Autodesk Fusion 360 part; units mm, degrees
sketch "Sketch1" plane through (0, 0, 0) normal (0, 1, 0) x (1, 0, 0)
  line L0 (4.25, 1.85) -> (-4.25, 1.85)
  line L1 (-4.25, 1.85) -> (-4.25, -1.85)
  line L2 (-4.25, -1.85) -> (4.25, -1.85)
  line L3 (4.25, -1.85) -> (4.25, 1.85)
  line L4 (4.25, 1.85) -> (-4.25, -1.85) construction
  line L5 (-4.25, 1.85) -> (4.25, -1.85) construction
  dimension "d1" = 8.5
  dimension "d2" = 3.7
extrude "Extrude1" add sketch "Sketch1" along normal blind 3.3
sketch "Sketch2" plane through (0, 3.3, 0) normal (0, 1, 0) x (-1, 0, 0)
  line L0 (-4.25, 1.85) -> (-4.25, -1.85)
  line L1 (-4.25, -1.85) -> (4.25, -1.85)
  line L2 (4.25, -1.85) -> (4.25, 1.85)
  line L3 (4.25, 1.85) -> (-4.25, 1.85)
  line L4 (-4.25, 0) -> (-1.75, 0)
  line L5 (-1.75, 0) -> (-1.1, 0)
  line L6 (-1.75, -0.65) -> (-0.45, -0.65)
  line L7 (-0.45, -0.65) -> (-0.45, 0.65)
  line L8 (-0.45, 0.65) -> (-1.75, 0.65)
  line L9 (-1.75, 0.65) -> (-1.75, -0.65)
  line L10 (-1.75, -0.65) -> (-0.45, 0.65) construction
  line L11 (-0.45, -0.65) -> (-1.75, 0.65) construction
  line L12 (4.25, 0) -> (1.75, 0)
  line L13 (1.75, 0) -> (1.1, 0)
  line L14 (0.45, -0.65) -> (1.75, -0.65)
  line L15 (1.75, -0.65) -> (1.75, 0.65)
  line L16 (1.75, 0.65) -> (0.45, 0.65)
  line L17 (0.45, 0.65) -> (0.45, -0.65)
  line L18 (0.45, -0.65) -> (1.75, 0.65) construction
  line L19 (1.75, -0.65) -> (0.45, 0.65) construction
  line L20 (0.45, -0.65) -> (-0.45, -0.65)
  line L21 (0.45, 0.65) -> (-0.45, 0.65)
  point P0 (-1.1, 0)
  point P1 (1.1, 0)
  dimension "d5" = 2.5
  dimension "d6" = 0.65
  dimension "d7" = 1.3
  dimension "d8" = 1.3
  dimension "d9" = 2.5
  dimension "d10" = 0.65
  dimension "d11" = 1.3
  dimension "d12" = 1.3
extrude "Extrude2" cut sketch "Sketch2" against normal blind 0.1 contours L14 L15 L16 L17 | L7 L17 L20 L21
extrude "Extrude3" add sketch "Sketch2" along normal blind 3 contours L6 L7 L8 L9
chamfer "Chamfer1" distance 0.2 angle 45 4 edges at (1.1, 6.3, 0.65) (0.45, 6.3, 0) (1.1, 6.3, -0.65) (1.75, 6.3, 0)
chamfer "Chamfer2" distance 0.1 angle 45 12 edges at (0, 3.3, 1.85) (4.25, 3.3, 0) (-4.25, 3.3, 0) (0, 3.3, -1.85) (4.25, 1.65, 1.85) (4.25, 1.65, -1.85) (4.25, 0, 0) (0, 0, 1.85) (-4.25, 1.65, 1.85) (-4.25, 1.65, -1.85) (0, 0, -1.85) (-4.25, 0, 0)
sketch "Sketch3" plane through (0, 0, 0) normal (0, -1, 0) x (1, 0, 0)
  line L0 (-4.15, -1.75) -> (4.15, -1.75)
  line L1 (4.15, -1.75) -> (4.15, 1.75)
  line L2 (4.15, 1.75) -> (-4.15, 1.75)
  line L3 (-4.15, 1.75) -> (-4.15, -1.75)
  line L4 (0.15, 0.1) -> (-0.15, 0.1)
  line L5 (-0.15, 0.1) -> (-0.15, -0.1)
  line L6 (-0.15, -0.1) -> (0.15, -0.1)
  line L7 (0.15, -0.1) -> (0.15, 0.1)
  line L8 (0.15, 0.1) -> (-0.15, -0.1) construction
  line L9 (-0.15, 0.1) -> (0.15, -0.1) construction
  line L10 (0, 0) -> (2.7, 0)
  line L11 (2.7, 0) -> (2.55, 0)
  line L12 (2.7, 0.1) -> (2.4, 0.1)
  line L13 (2.4, 0.1) -> (2.4, -0.1)
  line L14 (2.4, -0.1) -> (2.7, -0.1)
  line L15 (2.7, -0.1) -> (2.7, 0.1)
  line L16 (2.7, 0.1) -> (2.4, -0.1) construction
  line L17 (2.4, 0.1) -> (2.7, -0.1) construction
  line L18 (-0.15, 0) -> (-2.85, 0)
  line L19 (-2.85, 0) -> (-2.7, 0)
  line L20 (-2.55, 0.1) -> (-2.85, 0.1)
  line L21 (-2.85, 0.1) -> (-2.85, -0.1)
  line L22 (-2.85, -0.1) -> (-2.55, -0.1)
  line L23 (-2.55, -0.1) -> (-2.55, 0.1)
  line L24 (-2.55, 0.1) -> (-2.85, -0.1) construction
  line L25 (-2.85, 0.1) -> (-2.55, -0.1) construction
  point P0 (2.55, 0)
  point P1 (-2.7, 0)
  dimension "d19" = 0.3
  dimension "d20" = 0.2
  dimension "d23" = 2.7
  dimension "d24" = 0.15
  dimension "d25" = 0.3
  dimension "d26" = 0.2
  dimension "d27" = 2.7
  dimension "d28" = 0.15
  dimension "d29" = 0.3
  dimension "d30" = 0.2
extrude "Extrude4" add sketch "Sketch3" along normal blind 5 contours L4 L5 L6 L7
extrude "Extrude5" add sketch "Sketch3" along normal blind 5 contours L18 L19 L21 L22 L23 | L18 L19 L20 L21 L23
extrude "Extrude6" add sketch "Sketch3" along normal blind 5 contours L10 L11 L12 L13 L15 | L10 L11 L13 L14 L15
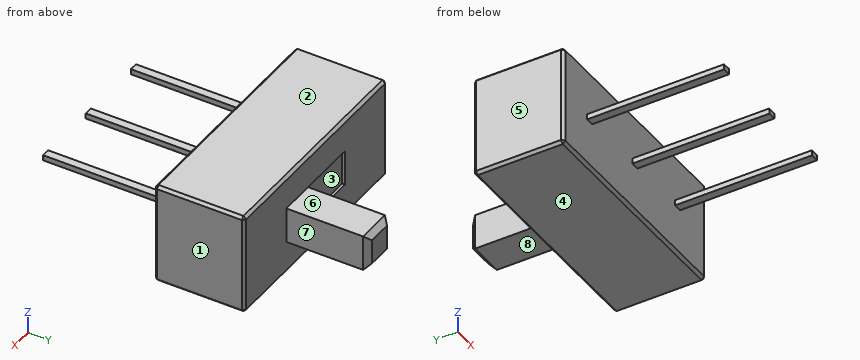
Input: part model. Units: mm. Frame: model coordinates. Face numbers are marked on the shaded views. A direction names the side the tool comes from. Coordinates: 2 decimals unless noted, no trailing zeros. Write each loop counter-clockwise with the first axis right and the second up, starting at its lowest first coordinate (ties: lowest second). Pieces come first, ordered by that corner, then holes. Notation, with made-up numbers: (-24.75, 58) -> (22.25, 58) arc R23 cw to (22.25, 70) -> close; hole circle Ø5 at (-11, -17.5). An arc over 180 degrees is marked (long way). Answer as a JSON object with one key per item and string values.
1. Section D-D on y = 5.25. Return the cut outline in (x, z), then the cut area to 3 significant figures.
Result set:
{"outline": "(0.45, -0.65) -> (1.75, -0.65) -> (1.75, 0.65) -> (0.45, 0.65) -> close", "area": "1.69 mm2"}
2. First-contact query: P1, Ø1, axis at y = 5, z = 0, coming from the +X side; P2, Ø0.6, axis at x = 1, y = 4.5, coming from the +Z side; P3, Ø0.6, axis at x = -0.5, z = 0, coming from the +Y side. Flat tips, straight axial feed; report the tip coordinate or a pass-through.
Result set:
{"P1": "stops at x = 1.75", "P2": "stops at z = 0.65", "P3": "stops at y = 3.2"}
3. Section A-A on y = -3. Return the cut outline in (x, z), then the cut area to 3 significant figures.
Result set:
{"outline": "(-2.85, -0.1) -> (-2.55, -0.1) -> (-2.55, 0.1) -> (-2.85, 0.1) -> close; (-0.15, -0.1) -> (0.15, -0.1) -> (0.15, 0.1) -> (-0.15, 0.1) -> close; (2.4, -0.1) -> (2.7, -0.1) -> (2.7, 0.1) -> (2.4, 0.1) -> close", "area": "0.180 mm2"}
4. Section C-C on z = -0.95. Return the cut outline in (x, y).
Result set:
{"outline": "(-4.25, 0.1) -> (-4.15, 0) -> (4.15, 0) -> (4.25, 0.1) -> (4.25, 3.2) -> (4.15, 3.3) -> (-4.15, 3.3) -> (-4.25, 3.2) -> close"}
5. Mould query, pull axis Z, two halves, no side actions, for the marked faces 1, 2, 3 and 4. Classes: released by +Z, released by -Z, zero draft, split by the parting line, or undercut.
Result set:
{"face 1": "zero draft", "face 2": "released by +Z", "face 3": "undercut", "face 4": "released by -Z"}
6. Access query for the marked faces 5, 6, 7 and 8. Directions: +Z, -Z, +X, -X, +Y, -Y. A direction counts if a zero-diameter tool reaches every point of the face in a straight line with its end or side. Return the directions, or none.
Result set:
{"face 5": "+Z, -Z, -X, +Y, -Y", "face 6": "+Z, +X, -X, +Y", "face 7": "+Z, -Z, +X, +Y", "face 8": "-Z, +X, -X, +Y"}
7. Section B-B on x = -1. Return the cut outline in (y, z), then the cut area to 3 significant figures.
Result set:
{"outline": "(0, -1.75) -> (0.1, -1.85) -> (3.2, -1.85) -> (3.3, -1.75) -> (3.3, -0.65) -> (3.2, -0.65) -> (3.2, 0.65) -> (3.3, 0.65) -> (3.3, 1.75) -> (3.2, 1.85) -> (0.1, 1.85) -> (0, 1.75) -> close", "area": "12.1 mm2"}
8. Material intervals for line 1 (Y direction, x = -2.75, z = -1.15); line 2 (Y direction, x = -1.25, z = -0.15); line 3 (X direction, y = 4, z = -0.15), sorted ascending. Write a range as from..to.
Result set:
{"line 1": "y = 0..3.3", "line 2": "y = 0..3.2", "line 3": "x = 0.45..1.75"}
